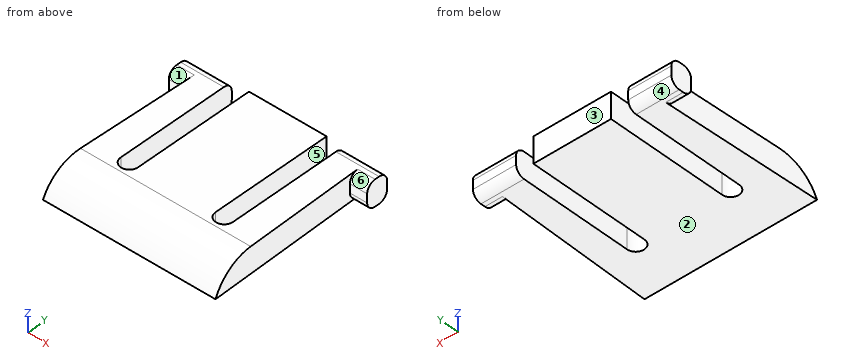
```python
from build123d import *

# Parameters (mm, degrees)
F4_DEPTH    = 3
F1_R        = 1
F3_T1_DEPTH = 42.9128784748


# Not quite as in the source:
# - a fillet or chamfer that OpenCascade refuses, or shapes differently, is made with other operations: its cross-section is extruded or revolved along the edge and cut away or added


with BuildPart() as f4:
    # F0 (on Top) → F4 (new body)
    with BuildSketch(Plane.XY):
        with BuildLine():
            Line((0, 20), (0, 0))
            Line((0, 0), (10, 0))
            Line((10, 0), (9.5, 17.5))
            Line((9.5, 17.5), (11.5, 17.5))
            Line((11.5, 17.5), (11.5, 20))
            Line((11.5, 20), (6.5, 20))
            Line((6.5, 20), (6.5, 6))
            ThreePointArc((6.5, 6), (5.5, 5), (4.5, 6))
            Line((4.5, 6), (4.5, 20))
            Line((4.5, 20), (0, 20))
        make_face()
    extrude(amount=F4_DEPTH)

    # F1
    f1_edges = [f4.edges().sort_by_distance(p)[0] for p in [
        (10.5, 17.5, 3),
        (9, 20, 3),
        (10.5, 17.5, 0),
        (9, 20, 0),
    ]]
    fillet(f1_edges, radius=F1_R)

    # F2: F4 across plane


with BuildPart() as f4_1:
    add(f4.part)
    add(f4.part.mirror(Plane.YZ))

    # F3: fillet of radius 5 on 1 edges, made by hand

    # F3_s2 → F3_t1 (cut)
    with BuildSketch(Plane.YZ.offset(-21.4564392374)):
        with BuildLine():
            ThreePointArc((4.582575695, 3), (1.8439629074, 2.1833001327), (0, 0))
            Line((0, 0), (0, 3))
            Line((0, 3), (4.582575695, 3))
        make_face()
    extrude(amount=F3_T1_DEPTH, mode=Mode.SUBTRACT)


solid = f4_1.part
```
Work out the finished part from the listing and answer in its coordinate system (mm). Face numbers are marked on the shaded views. A direction names the side the tool comes from. Give positions to 0.01 mm unless a question says otherwise; leave off trailing zeros. Loops run counter-clockwise (first coordinate to the right, second up) from the corner with the lowest first, then second, coordinate; pieces in that order, holes last. Notation, with made-up numbers: (64, 11) -> (122, 11) arc R24 cw to (122, 29) -> close; hole circle Ø9 at (-27.5, 2). An arc over 180 degrees is marked (long way). Put each result on its own line as item: value. Start each with the question number.
Item 1: Which of the six approach directions +Z, -Z, +X, -X, +Y, -Y give full straight-line access (tool end or side, diameter ignored) to the marked faces 4, 5 and 6?
Item 2: The part is cut by section B-B (x = 8.75). Give the vertices of the cut face in (y, z), then the cut area to 3 significant figures.
Item 3: The part is cut by section C-C (z = 2.5). Give the vertices of the cut face in (x, y).
Item 4: Find the intervals of material crossed by L1, parallel to X at y = 18.25, z = 1; L2, parallel to X at y = 14, z = 2.3; L3, parallel to Y at x = -7.75, z = 0.55, in increasing order. Write a range as [from, to].
Item 5: The part is cut by section D-D (y = 8.25). Give the vertices of the cut face in (x, z).
Item 6: The part is cut by section A-A (y = 15.75). Give the vertices of the cut face in (x, z).
Item 7: Each of these flat-tipped pins is pushed along its axis until it touches: P1, Ø0.5, axis at x = 10, z = 1.5, coming from the -Y side; P2, Ø1, axis at y = 5.5, z = 0.5, coming from the +X side; P3, Ø0.9, axis at y = 14.5, z = 1, coming from the +X side; P4, Ø5, axis at x = 7, y = 3.5, coming from the -Z side. Where does it stop, or does it pass through?
Item 8: The mould has two halves that part along Y. Classify the marked faces 1, 2 and 3: released by +Y, released by -Y, zero draft, split by the parting line, or undercut.
Answers below:
1. face 4: -Z, -X, +Y
1. face 5: +Z, -Z, +Y
1. face 6: +Z, +X
2. outline: (0, 0) -> (19, 0) arc R1 ccw to (20, 1) -> (20, 2) arc R1 ccw to (19, 3) -> (4.58, 3) arc R5 ccw to start
2. area: 55.7 mm2
3. outline: (-11.5, 17.63) -> (-9.5, 17.63) -> (-9.93, 2.4) -> (9.93, 2.4) -> (9.5, 17.63) -> (11.5, 17.63) -> (11.5, 19.87) -> (6.5, 19.87) -> (6.5, 6) arc R1 cw to (4.5, 6) -> (4.5, 20) -> (-4.5, 20) -> (-4.5, 6) arc R1 cw to (-6.5, 6) -> (-6.5, 19.87) -> (-11.5, 19.87) -> close
4. L1: [-11.5, -6.5], [-4.5, 4.5], [6.5, 11.5]
4. L2: [-9.6, -6.5], [-4.5, 4.5], [6.5, 9.6]
4. L3: [0.28, 19.89]
5. outline: (-9.76, 0) -> (-6.5, 0) -> (-6.5, 3) -> (-9.76, 3) -> close; (-4.5, 0) -> (4.5, 0) -> (4.5, 3) -> (-4.5, 3) -> close; (6.5, 0) -> (9.76, 0) -> (9.76, 3) -> (6.5, 3) -> close
6. outline: (-9.55, 0) -> (-6.5, 0) -> (-6.5, 3) -> (-9.55, 3) -> close; (-4.5, 0) -> (4.5, 0) -> (4.5, 3) -> (-4.5, 3) -> close; (6.5, 0) -> (9.55, 0) -> (9.55, 3) -> (6.5, 3) -> close
7. P1: y = 0.78
7. P2: x = 9.86
7. P3: x = 9.6
7. P4: z = 0
8. face 1: undercut
8. face 2: zero draft
8. face 3: released by +Y
